Could you check a few things on this model? Use its own coordinates, in mm. A direction names the side the tool comes from. Coordinates: 2 decimals unless noted, no trailing zeros. Write each loop counter-clockwise with the first axis right and the second up, starting at its lowest first coordinate (ties: lowest second). Pieces come first, ordered by that corner, then holes. Notation, with made-up numbers: M 5,17.5 L 61,17.5 A19 ccw 61,21.5 Z; hole C 56.5,63 d11. An arc over 180 degrees is marked long. Answer as CSV lines item,"result". Start each with the question number.
Item 1: Suppose I cut it at B-B, the plane x = 37. Write out the boundary of the cut face in (y, z).
Item 2: Suppose I cut it at D-D, the plane y = 0. State how many separate pieces and enclosed holes the cut face has, and give its area (3 significant figures).
Item 3: We'd pull the mould along X, two halves only. Please class faces 1 (the cylindrical face through (16.524, 16.71, -0.986)), 2 (the cylindrical face through (-16.524, -16.71, -0.986)), 3 (the cylindrical face through (2.17, -9.76, 14.76)), 4 (the flat face through (9, 31, 17)): +X half, -X half, draft (parallel to the pull), parting line (faces both ways), or undercut.
Item 4: Suppose I cut it at C-C, the plane y = 20. Write out the boundary of the cut face in (x, z), and give its area (3 significant figures).
Item 5: Suppose I cut it at A-A, the plane z = 24. Write out the boundary of the cut face in (x, y).
Item 6: I'm going to push flat-ended pins straight in: P1, Ø9.5, axis at x = -20, y = 0, coming from the +Z side; P2, Ø1, axis at x = 32.5, z = 11.5, coming from the -Y side; P3, Ø2, axis at x = 1.5, y = -13, coming from the -Z side; P4, Ø9, axis at x = -37, y = 0, coming from the -Z side. Where does each tip first touch, or does it pass through?
Item 7: On a 3-axis mill with a long thin cutter (end or side, diameter ignored), from which of +Z, -Z, +X, -X, +Y, -Y can I reach the whole of each face in a straight line? I mean faces 5 (the cylindrical face through (-4.036, 30.736, 24.395)), 6 (the cylindrical face through (-11, 0, 5)), 7 (the cylindrical face through (16.71, -16.524, -0.986)), 8 (the cylindrical face through (0.44, -40.37, 8.62)). Say none if no direction works.
Item 8: If I drill on line 1 along Y through (x, z) = (0, 6); line 2 along Z through (x, y) = (-23.5, 35); line 3 along Y through (x, z) = (15, 7), over which ranges is the centre line in solid material (lowest first)? Write a range as [from, to].
```python
from build123d import *

# Parameters (mm, degrees)
F0_R     = 45
F1_DEPTH = 17
F2_R     = 31
F3_DEPTH = 15
F6_R     = 23.5
F7_DEPTH = 2
F9_D     = 18
F9_DEPTH = 13.5
F9_TIP   = 5.4077455712
F10_D    = 20
F11_D    = 10.5
F13_D    = 6.8


with BuildPart() as f1:
    # F0 (on Top) → F1 (new body)
    with BuildSketch(Plane.XY):
        Circle(F0_R)
    extrude(amount=F1_DEPTH)

    # F2 (on face) → F3 (join)
    with BuildSketch(Plane.XY.offset(17)):
        Circle(F2_R)
    extrude(amount=F3_DEPTH)

    # F6 (on face) → F7 (join)
    with BuildSketch(Plane(origin=(0, 0, 0), x_dir=(1, 0, 0), z_dir=(0, 0, -1))):
        Circle(F6_R)
    extrude(amount=F7_DEPTH)

    # F9
    with Locations(Plane(origin=(0, 0, -2), x_dir=(1, 0, 0), z_dir=(0, 0, -1))):
        with Locations((-20, 0), (0, 20), (20, 0), (0, -20)):
            Hole(F9_D / 2, depth=F9_DEPTH)
            with Locations((0, 0, -(F9_DEPTH + F9_TIP / 2))):  # 118° drill point
                Cone(0, F9_D / 2, F9_TIP, mode=Mode.SUBTRACT)

    # F10 (through all)
    with Locations(Plane.XY.offset(32)):
        with Locations((0, 0)):
            Hole(F10_D / 2)

    # F11 (through all)
    with Locations(Plane.XY.offset(32)):
        with Locations((-20, 0), (0, 20), (20, 0), (0, -20)):
            Hole(F11_D / 2)

    # F13 (through all)
    with Locations(Plane(origin=(0, 0, 0), x_dir=(1, 0, 0), z_dir=(0, 0, -1))):
        with Locations((0, 37), (-37, 0), (0, -37), (37, 0)):
            Hole(F13_D / 2)


solid = f1.part
```
Ans:
1,outline,"M -25.61,0 L -3.4,0 L -3.4,17 L -25.61,17 Z; M 3.4,0 L 25.61,0 L 25.61,17 L 3.4,17 Z"
2,separate pieces,"6"
2,enclosed holes,"0"
2,area,"731 mm^2"
3,face 1,"+X half"
3,face 2,"-X half"
3,face 3,"undercut"
3,face 4,"draft"
4,outline,"M -40.31,0 L -12.34,0 L -12.34,-2 L -9,-2 L -9,11.5 L -5.25,13.75 L -5.25,32 L -23.69,32 L -23.69,17 L -40.31,17 Z; M 5.25,13.75 L 9,11.5 L 9,-2 L 12.34,-2 L 12.34,0 L 40.31,0 L 40.31,17 L 23.69,17 L 23.69,32 L 5.25,32 Z"
4,area,"1,660 mm^2"
5,outline,"C 0,0 d62; hole C -20,0 d10.5; hole C 0,0 d20; hole C 0,-20 d10.5; hole C 0,20 d10.5; hole C 20,0 d10.5"
6,P1,"passes through"
6,P2,"stops at y = -31.64"
6,P3,"stops at z = 12.01"
6,P4,"stops at z = 0"
7,face 5,"+Z"
7,face 6,"-Z"
7,face 7,"-Z, +X, -Y"
7,face 8,"+Z, -Z"
8,line 1,"y = [-45, -40.4], [-33.6, -29], [-11, -10], [10, 11], [29, 33.6], [40.4, 45]"
8,line 2,"z = [0, 17]"
8,line 3,"y = [-42.43, -7.48], [7.48, 42.43]"
